from build123d import *

# Parameters (mm, degrees)
F4_DEPTH      = 3.175
F7_DEPTH      = 42.545
F7_DEPTH_BACK = 42.545
F8_R          = 12.7
F9_DEPTH      = 42.545
F9_DEPTH_BACK = 42.545


with BuildPart() as f1:
    # F0 (on Front) → F1 (revolve)
    with BuildSketch(Plane.XZ):
        with BuildLine():
            ThreePointArc((0, 101.6), (-25.7938219347, 88.3632722661), (-30.0805069771, 59.69))
            Line((-30.0805069771, 59.69), (-6.35, 48.6774114908))
            Line((-6.35, 48.6774114908), (-6.35, 12.7))
            Line((-6.35, 12.7), (-30.0805069771, 12.7))
            Line((-30.0805069771, 12.7), (-30.0805069771, 47.3746955395))
            Line((-30.0805069771, 47.3746955395), (-35.56, 47.3746955395))
            Line((-35.56, 47.3746955395), (-35.56, 0))
            Line((-35.56, 0), (0, 0))
            Line((0, 0), (35.56, 0))
            Line((35.56, 0), (35.56, 47.3746955395))
            Line((35.56, 47.3746955395), (30.0805069771, 47.3746955395))
            Line((30.0805069771, 47.3746955395), (30.0805069771, 12.7))
            Line((30.0805069771, 12.7), (6.35, 12.7))
            Line((6.35, 12.7), (6.35, 48.6774114908))
            Line((6.35, 48.6774114908), (30.0805069771, 59.69))
            ThreePointArc((30.0805069771, 59.69), (25.7938219347, 88.3632722661), (0, 101.6))
        make_face()
    revolve(axis=Axis((17.78, 0, 0), (-1, 0, 0)))



with BuildPart() as f4:
    # F3 (on offset) → F4 (new body)
    with BuildSketch(Plane.YZ.offset(45.72)):
        with BuildLine():
            Line((22.8975321566, -10.9937719249), (95.25, 139.7))
            Line((95.25, 139.7), (-95.25, 139.7))
            Line((-95.25, 139.7), (-22.8975321566, -10.9937719249))
            ThreePointArc((-22.8975321566, -10.9937719249), (0, -25.4), (22.8975321566, -10.9937719249))
        make_face()
    extrude(amount=-F4_DEPTH)


with BuildPart() as f5_1:
    # F5: instance of F4
    add(f4.part.mirror(Plane.YZ))


with BuildPart() as f4_1:
    add(f4.part)

    add(f5_1.part)  # F7 merges F5_1
    # F6 (on Right) → F7 (join, two sides)
    with BuildSketch(Plane.YZ) as f7_sk:
        Polygon((95.25, 139.7), (-95.25, 139.7), (-93.7255900495, 136.525), (93.7255900495, 136.525), align=None)
    extrude(amount=F7_DEPTH)
    extrude(f7_sk.sketch, amount=-F7_DEPTH_BACK)


with BuildPart() as f1_1:
    add(f1.part)

    add(f4_1.part)  # F9 merges F4
    # F8 (on Right) → F9 (join, two sides)
    with BuildSketch(Plane.YZ) as f9_sk:
        Circle(F8_R)
    extrude(amount=F9_DEPTH)
    extrude(f9_sk.sketch, amount=-F9_DEPTH_BACK)


solid = f1_1.part
The model under review builds one solid part; all positions refer to its coordinate system, in mm. A direction names the side the tool comes from. Round coordinates to 2 decimals unless told otherwise and drop trailing zeros. Write each loop counter-clockwise with the first axis right and the second up, starting at its lowest first coordinate (ties: lowest second). Pieces come first, ordered by that corner, then holes. Notation, with made-up numbers: M -7.5,-26.5 L 27.5,-26.5 A36 ccw 27.5,9.5 Z; hole C 85,37.5 d5. An arc over 180 degrees is marked long. Use a Markdown table: item, result. Add a question column.
Q1. Machinability: for faces 1 (the face through (-30.081, -10, -10)), 2 (the face through (44.155, -0.399, -25.397)), 3 (the face through (1, -1, 136.525)), which of the approach directions +Z, -Z, +X, -X, +Y, -Y give a long, thin tool a straight path to every point of the face, cutting with its end or side? Answer none if there is none.
Q2. We need section A-A, the plane x = 26. State the section outline as (y, z) points (3 decimals).
Q3. The part is to be moulded in two halves that separate along Z. For faces 4 (the face through (-45.72, -1, 77)), 5 (the face through (1, 1, 139.7)), 6 (the face through (-44.155, -0.399, -25.397)), 7 (the face through (-42.545, -1, 75)), say which applies: pulls with the +Z half, pulls with the -Z half, needs draft (parallel to the pull), parting line crosses it, or undercut.
Q4. We need section B-B, the plane y = 40. Count the separate pieces of the cut face and the enclosed holes in it, plus the area to 3 significant figures.
Q5. Insertion check: pin 1 (6 mm diameter, centred on y = 79, z = 98, fed in from +X); pin 2 (4 mm diameter, centred on y = 22.5, z = -20.5, fed in from -X); pin 3 (5 mm diameter, centred on x = 27.5, y = 18.5, fed in from -Z); pin 4 (6 mm diameter, centred on x = 8.5, z = 40.5, fed in from +Y). Each pin has a flat end and moves straight along its axis. Give the tip position at first contact, or say it passes through.
Q6. To check wall thickness, follow line 1 (X direction, y = -34.5, z = -16); line 2 (Z direction, x = -15, y = -37.5) (3 decimals); line 3 (X direction, y = 87, z = 127.5) (3 decimals). State the ranges of each line that lie inside material, in increasing order.
Findings below:
| question | item | result |
|---|---|---|
| 1 | face 1 | none |
| 1 | face 2 | -Z, +X |
| 1 | face 3 | +Y, -Y |
| 2 | outline | M -95.25,139.7 L -93.726,136.525 L 93.726,136.525 L 95.25,139.7 Z; C 0,0 d176.145; C 0,0 d25.4; hole C 0,0 d115.593 |
| 3 | face 4 | needs draft |
| 3 | face 5 | pulls with the +Z half |
| 3 | face 6 | pulls with the -Z half |
| 3 | face 7 | undercut |
| 4 | separate pieces | 4 |
| 4 | enclosed holes | 0 |
| 4 | area | 8,680 mm² |
| 5 | pin 1 | passes through |
| 5 | pin 2 | stops at x = -35.56 |
| 5 | pin 3 | stops at z = -87.53 |
| 5 | pin 4 | stops at y = 93.42 |
| 6 | line 1 | x = -35.56 to -30.08, -6.35 to 6.35, 30.08 to 35.56 |
| 6 | line 2 | z = -90.361 to -37.016, 37.016 to 90.361, 136.525 to 139.7 |
| 6 | line 3 | x = -45.72 to -42.545, 42.545 to 45.72 |
